Source: three-view drawing plus pictorial views. Frame: mm from the lowest corner of the part. A direction names the side the tool comes from. Give positions to 0.01 mm unless a question says otherwise; leave off trailing zeros. Loops run counter-clockwise (first coordinate to the right, second up) from the corner with the lowest first, then second, coordinate; pieces in that order, holes last. Notation, with made-up numbers: M 51.5,43 L 103.5,43 A9 ccw 103.5,50 Z; hole C 87.5,80.25 d8. An arc over 180 degrees is marked long. Write item = value, one per line.
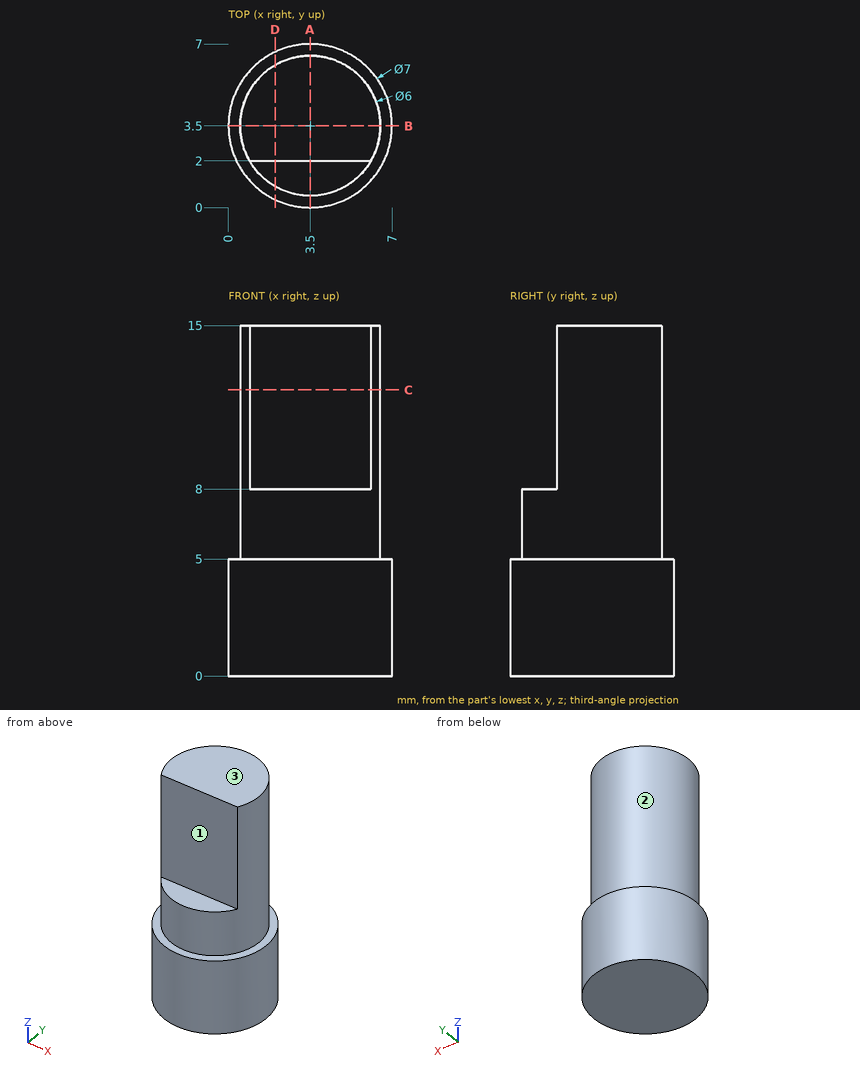
1. Reachability of the marked faces 1, 2 and 3 from +Z, -Z, +X, -X, +Y, -Y: full face, straight path, thin tool, end or side. Return the list, or none.
Derived:
face_1 = +Z, +X, -X, -Y
face_2 = +Z
face_3 = +Z, +X, -X, +Y, -Y
2. Material intervals for probe 1 along Z at (x, y) = (6.25, 5.5); probe 2 along Y at (x, z) = (5, 9.5); probe 3 along Y at (x, z) = (3, 10), sorted ascending. Write a range as from..to.
Derived:
probe_1 = 0..5
probe_2 = 2..6.1
probe_3 = 2..6.46
3. Cut plane A-A, the plane x = 3.5. Return the cut outline in (y, z), then the cut area to 3 significant figures.
Derived:
outline = M 0,0 L 7,0 L 7,5 L 6.5,5 L 6.5,15 L 2,15 L 2,8 L 0.5,8 L 0.5,5 L 0,5 Z
area = 84.5 mm²
4. Cut plane B-B, the plane y = 3.5. Return the cut outline in (x, z).
Derived:
outline = M 0,0 L 7,0 L 7,5 L 6.5,5 L 6.5,15 L 0.5,15 L 0.5,5 L 0,5 Z
5. Cut plane C-C, the plane z = 12.25. Return the cut outline in (x, y).
Derived:
outline = M 0.9,2 L 6.1,2 A3 ccw long Z
6. Cut plane D-D, the plane x = 2. Return the cut outline in (y, z).
Derived:
outline = M 0.34,0 L 6.66,0 L 6.66,5 L 6.1,5 L 6.1,15 L 2,15 L 2,8 L 0.9,8 L 0.9,5 L 0.34,5 Z
7. First-contact query: pin 1 Ø2 at (x, y) = (1.5, 5) entering from -Z; pin 2 Ø1.5 at (x, z) = (3.5, 11) entering from +Y; pin 3 Ø1.7 at (x, y) = (3.5, 1) entering from +Z; pin 4 Ø1.5 at (y, z) = (4, 11) entering from +X. Flat tips, straight axial feed; report the tip coordinate or a pass-through.
Derived:
pin_1 = 0
pin_2 = 6.5
pin_3 = 8
pin_4 = 6.5
